Part model, mm, in its own coordinate system. A direction names the side the tool comes from. Round coordinates to 2 decimals unless told otherwise and drop trailing zeros. Order: outer loops, then holes, each group sorted by start corner. A loop starts at its lowest first (then second) coordinate and runs counter-clockwise, first axis right, second up. Notation, with made-up numbers: M 89.25,73.5 L 94.25,73.5 A13 cw 94.25,82.5 Z; hole C -13,-35.75 d10. An arc over 180 degrees is marked long. Write each question's results on one line, items separated by ' | '. Start each with the question number.
1. Band-saw the part on B-B, the plane z = 21. List the corners of the cut face in (x, y).
2. Drop a flat-ended pin along its axis: pin 1 Ø4 at (x, z) = (35.5, 10) entering from -Y. Give the stop position or say it passes through.
3. Band-saw the part on D-D, the plane x = 20. List the corners of the cut face in (y, z), then the cut area to 3 significant figures.
4. Probe L1, parallel to Y at x = 38, z = 14.75; L2, parallel to Y at x = 29.5, z = 2; L3, parallel to X at y = -17, z = 19.5 (3 decimals). List the from-to ranges inside material, lowest first. Write a range as [from, to].
5. Which spindle directions (+Z, -Z, +X, -X, +Y, -Y) get a long thin tool onto all of the face, cutting with end or side? Do faces 1 (the face through (25.3, -31.8, 12.9)), 2 (the face through (22.27, -6.26, 12.52)), 3 (the face through (0, -19, 13)). Say none if no direction does.
6. Band-saw the part on A-A, the plane x = 26.5. List the corners of the cut face in (y, z), then the cut area to 3 significant figures.
7. Band-saw the part on C-C, the plane y = -23.5. List the corners of the cut face in (x, z).
```python
from build123d import *

# Parameters (mm, degrees)
F0_W     = 50.8
F0_H     = 25.4
F1_DEPTH = 38.1
F3_DEPTH = 12.7
F5_DEPTH = 25.4
F7_DEPTH = 12.7


with BuildPart() as f1:
    # F0 (on Front) → F1 (new body)
    with BuildSketch(Plane.XZ):
        with Locations((25.4, 12.7)):
            Rectangle(F0_W, F0_H)
    extrude(amount=F1_DEPTH)

    # F2 (on face) → F3 (cut)
    with BuildSketch(Plane.XZ.offset(38.1)):
        Polygon((19.05, 25.4), (31.75, 0), (50.8, 0), (50.8, 25.4), align=None)
    extrude(amount=-F3_DEPTH, mode=Mode.SUBTRACT)

    # F4 (on face) → F5 (cut)
    with BuildSketch(Plane.XZ.offset(25.4)):
        Polygon((50.8, 25.4), (44.45, 25.4), (50.8, 0), align=None)
    extrude(amount=-F5_DEPTH, mode=Mode.SUBTRACT)

    # F6 (on face) → F7 (cut)
    with BuildSketch(Plane(origin=(0, 0, 0), x_dir=(-1, 0, 0), z_dir=(0, 1, 0))):
        Polygon((-50.8, 0), (-25.4, 0), (-19.05, 25.4), (-44.45, 25.4), align=None)
    extrude(amount=-F7_DEPTH, mode=Mode.SUBTRACT)


solid = f1.part
```
Solution:
1) outline: M 0,-38.1 L 21.25,-38.1 L 21.25,-25.4 L 45.55,-25.4 L 45.55,-12.7 L 20.15,-12.7 L 20.15,0 L 0,0 Z
2) pin 1: y = -25.4
3) outline: M -38.1,0 L 0,0 L 0,21.6 L -12.7,21.6 L -12.7,25.4 L -25.4,25.4 L -25.4,23.5 L -38.1,23.5 Z | area: 895 mm^2
4) L1: [-25.4, -12.7] | L2: [-38.1, -12.7] | L3: [0, 45.925]
5) face 1: +Z, +X, -Y | face 2: +Z, +X, +Y | face 3: +Z, -Z, -X, +Y, -Y
6) outline: M -38.1,0 L -12.7,0 L -12.7,25.4 L -25.4,25.4 L -25.4,10.5 L -38.1,10.5 Z | area: 456 mm^2
7) outline: M 0,0 L 50.8,0 L 44.45,25.4 L 0,25.4 Z
